```python
from build123d import *

# Parameters (mm, degrees)
F0_W      = 390
F0_H      = 490
F0_W_2    = 127.5
F0_H_2    = 400
F1_DEPTH  = 45
F2_W      = 45
F2_H      = 45
F3_DEPTH  = 200
F4_W      = 45
F4_H      = 45
F5_DEPTH  = 45
F6_W      = 45
F6_H      = 45
F7_DEPTH  = 445
F8_W      = 12
F8_H      = 45
F9_DEPTH  = 10
F10_W     = 12
F10_H     = 45
F11_DEPTH = 10
F13_DEPTH = 35
F15_DEPTH = 12
F16_W     = 12
F16_H     = 45
F17_DEPTH = 10
F18_W     = 12
F18_H     = 45
F19_DEPTH = 10
F21_DEPTH = 35
F23_DEPTH = 12
F24_W     = 45
F24_H     = 30
F25_DEPTH = 30
F26_W     = 30
F26_H     = 30
F27_DEPTH = 27.5
F28_W     = 30
F28_H     = 30
F29_DEPTH = 27.5


with BuildPart() as f1:
    # F0 (on Top) → F1 (new body)
    with BuildSketch(Plane.XY):
        with Locations((195, 245)):
            Rectangle(F0_W, F0_H)
        with Locations((108.75, 245)):
            Rectangle(F0_W_2, F0_H_2, mode=Mode.SUBTRACT)
        with Locations((281.25, 245)):
            Rectangle(F0_W_2, F0_H_2, mode=Mode.SUBTRACT)
    extrude(amount=F1_DEPTH)

    # F2 (on face) → F3 (join)
    with BuildSketch(Plane.XY.offset(45)):
        with Locations((22.5, 22.5)):
            Rectangle(F2_W, F2_H)
        with Locations((22.5, 467.5)):
            Rectangle(F2_W, F2_H)
    extrude(amount=F3_DEPTH)

    # F4 (on face) → F5 (join)
    with BuildSketch(Plane(origin=(0, 0, 0), x_dir=(0, -1, 0), z_dir=(-1, 0, 0))):
        with Locations((-467.5, 177.5)):
            Rectangle(F4_W, F4_H)
    extrude(amount=F5_DEPTH)

    # F6 (on face) → F7 (join)
    with BuildSketch(Plane.XZ.offset(-445)):
        with Locations((-22.5, 177.5)):
            Rectangle(F6_W, F6_H)
    extrude(amount=F7_DEPTH)

    # F8 (on face) → F9 (join)
    with BuildSketch(Plane.YZ.offset(217.5)):
        with Locations((101, 22.5)):
            Rectangle(F8_W, F8_H)
    extrude(amount=F9_DEPTH)

    # F10 (on face) → F11 (join)
    with BuildSketch(Plane(origin=(172.5, 0, 0), x_dir=(0, -1, 0), z_dir=(-1, 0, 0))):
        with Locations((-101, 22.5)):
            Rectangle(F10_W, F10_H)
    extrude(amount=F11_DEPTH)

    # F12 (on face) → F13 (join)
    with BuildSketch(Plane.XY.offset(45)):
        Polygon((217.5, 95), (227.5, 95), (227.5, 107), (217.5, 107), (172.5, 107), (162.5, 107), (162.5, 95), (172.5, 95), align=None)
    extrude(amount=F13_DEPTH)

    # F14 (on face) → F15 (cut)
    with BuildSketch(Plane(origin=(0, 107, 0), x_dir=(-1, 0, 0), z_dir=(0, 1, 0))):
        Polygon((-172.5, 80), (-217.5, 80), (-195, 55), align=None)
    extrude(amount=-F15_DEPTH, mode=Mode.SUBTRACT)

    # F16 (on face) → F17 (join)
    with BuildSketch(Plane.YZ.offset(217.5)):
        with Locations((389, 22.5)):
            Rectangle(F16_W, F16_H)
    extrude(amount=F17_DEPTH)

    # F18 (on face) → F19 (join)
    with BuildSketch(Plane(origin=(172.5, 0, 0), x_dir=(0, -1, 0), z_dir=(-1, 0, 0))):
        with Locations((-389, 22.5)):
            Rectangle(F18_W, F18_H)
    extrude(amount=F19_DEPTH)

    # F20 (on face) → F21 (join)
    with BuildSketch(Plane.XY.offset(45)):
        Polygon((227.5, 383), (227.5, 395), (217.5, 395), (172.5, 395), (162.5, 395), (162.5, 383), (172.5, 383), (217.5, 383), align=None)
    extrude(amount=F21_DEPTH)

    # F22 (on face) → F23 (cut)
    with BuildSketch(Plane.XZ.offset(-383)):
        Polygon((217.5, 80), (172.5, 80), (195, 55), align=None)
    extrude(amount=-F23_DEPTH, mode=Mode.SUBTRACT)

    # F24 (on face) → F25 (join)
    with BuildSketch(Plane.XY.offset(200)):
        with Locations((-22.5, 180)):
            Rectangle(F24_W, F24_H)
        with Locations((-22.5, 310)):
            Rectangle(F24_W, F24_H)
    extrude(amount=F25_DEPTH)

    # F26 (on face) → F27 (join)
    with BuildSketch(Plane.YZ):
        with Locations((310, 215)):
            Rectangle(F26_W, F26_H)
        with Locations((180, 215)):
            Rectangle(F26_W, F26_H)
    extrude(amount=F27_DEPTH)

    # F28 (on face) → F29 (join)
    with BuildSketch(Plane(origin=(-45, 0, 0), x_dir=(0, -1, 0), z_dir=(-1, 0, 0))):
        with Locations((-310, 215)):
            Rectangle(F28_W, F28_H)
        with Locations((-180, 215)):
            Rectangle(F28_W, F28_H)
    extrude(amount=F29_DEPTH)


solid = f1.part
```
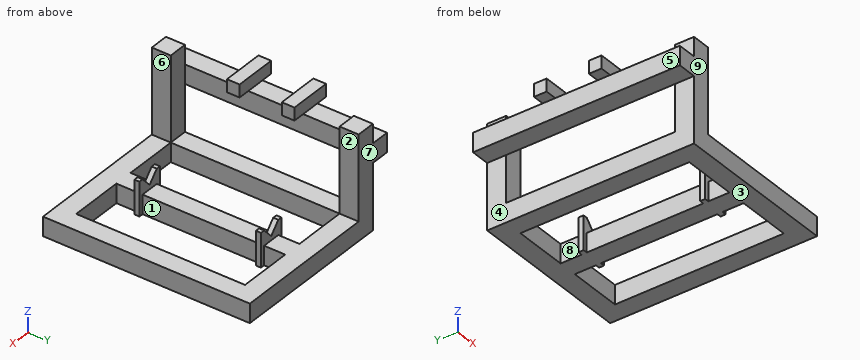
Verification items for the finished model (mm, model axes). Face numbers are marked on the shaded views. A direction names the side the tool comes from. Coordinates: 2 decimals unless noted, no trailing zeros. Loops run counter-clockwise (first coordinate to the right, second up) from the corner with the lowest first, then second, coordinate; pieces in that order, holes last. Notation, with made-up numbers: (59, 23.5) - (97, 23.5) arc R18 cw to (97, 31.5) - close; hole circle Ø7 at (10.5, 82). An arc over 180 degrees is marked (long way). Put each result on its own line as item: value.
Item 1: Section check D-D (z = 109.5). Enter the section's corners in (x, y), then the cut area to 3 significant figures.
Conclusion:
outline: (0, 0) - (45, 0) - (45, 45) - (0, 45) - close; (0, 445) - (45, 445) - (45, 490) - (0, 490) - close
area: 4,050 mm2
Item 2: Set-up check for the marked faces 5, 6, 7, 8 and 9: record each of +Z, -Z, +X, -X, +Y, -Y from which the full face is reachable in a straight line by a thin tool's end or side.
Conclusion:
face 5: -Z, -X, +Y, -Y
face 6: +Z, +X, +Y, -Y
face 7: +Z, -Z, +X, -X, +Y
face 8: +Z, -Z
face 9: +Z, -Z, +X, -X, -Y
Item 3: Section check B-B (x = 149.5). Enter the section's corners in (y, z), then the cut area to 3 significant figures.
Conclusion:
outline: (0, 0) - (45, 0) - (45, 45) - (0, 45) - close; (445, 0) - (490, 0) - (490, 45) - (445, 45) - close
area: 4,050 mm2
Item 4: Section check A-A (z = 206). Enter the section's corners in (x, y), then the cut area to 4 significant figures.
Conclusion:
outline: (-72.5, 165) - (27.5, 165) - (27.5, 195) - (-72.5, 195) - close; (-72.5, 295) - (27.5, 295) - (27.5, 325) - (-72.5, 325) - close; (0, 0) - (45, 0) - (45, 45) - (0, 45) - close; (0, 445) - (45, 445) - (45, 490) - (0, 490) - close
area: 10,050 mm2
Item 5: Draft check along X on the marked faces 1, 2, 3 and 4. Enter one of: pulls with the +X half, pulls with the -X half, needs draft (parallel to the pull), parting line crosses it, or undercut.
Conclusion:
face 1: undercut
face 2: pulls with the +X half
face 3: needs draft
face 4: pulls with the -X half
Item 6: Scan lines: line 1 along X through (y, z) = (78, 21); line 2 along Z through (x, y) = (14, 301); line 3 along X through (y, z) = (106, 30). Record each from-to range of solid material in increasing order.
Conclusion:
line 1: x = 0 to 45, 172.5 to 217.5, 345 to 390
line 2: z = 0 to 45, 200 to 230
line 3: x = 0 to 45, 162.5 to 227.5, 345 to 390
Item 7: Section check C-C (y = 434.5). Enter the section's corners in (x, z).
Conclusion:
outline: (-45, 155) - (0, 155) - (0, 200) - (-45, 200) - close; (0, 0) - (45, 0) - (45, 45) - (0, 45) - close; (172.5, 0) - (217.5, 0) - (217.5, 45) - (172.5, 45) - close; (345, 0) - (390, 0) - (390, 45) - (345, 45) - close
Item 8: Gauge pin test, flat ends, axial feed: pin 1 Ø3 at (y, z) = (110, 155) entering from +X; pin 2 Ø5 at (x, y) = (166, 99) entering from +Z; pin 3 Ø22 at (x, y) = (-55, 310) entering from -Z. Record the tip position at first contact, or that the pin passes through.
Conclusion:
pin 1: stops at x = 0
pin 2: stops at z = 80
pin 3: stops at z = 155
